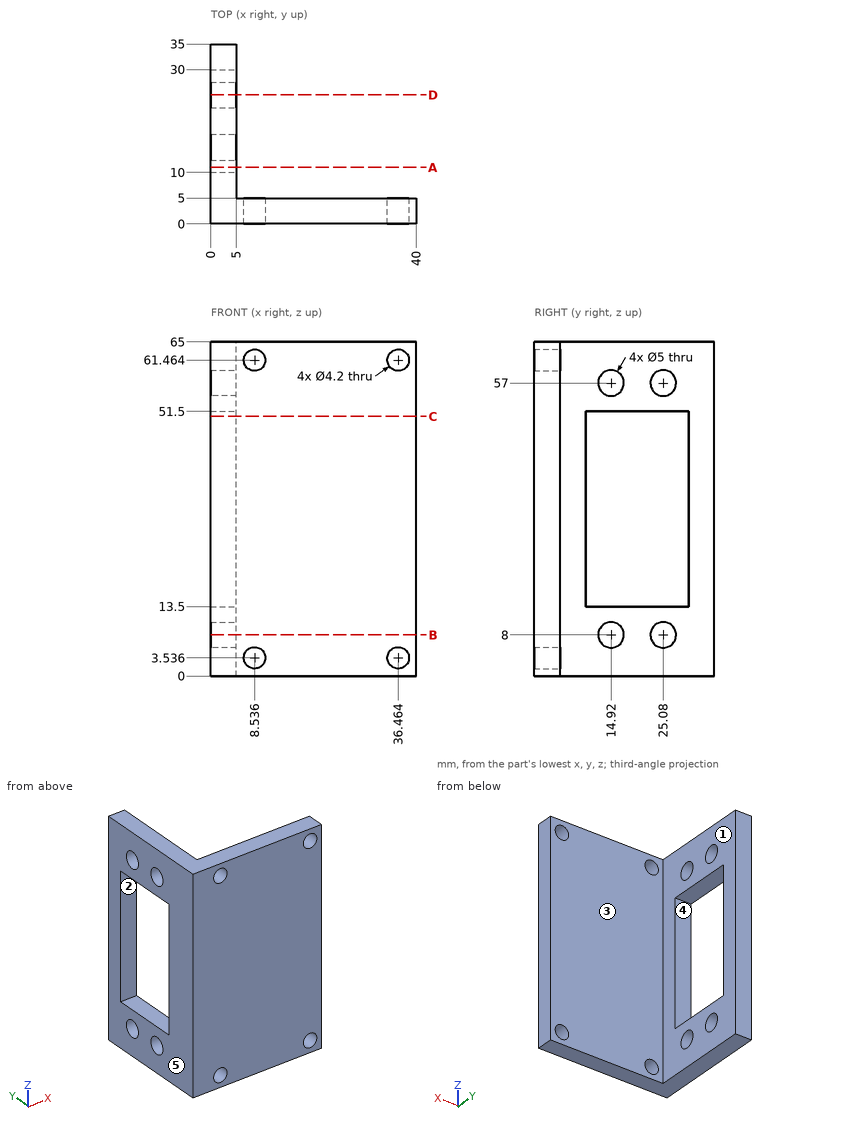
Source: three-view drawing plus pictorial views. Frame: mm from the lowest corner of the part. A direction names the side the tool comes from. Coordinates: 2 decimals unless noted, no trailing zeros. Loops run counter-clockwise (first coordinate to the right, second up) from the corner with the lowest first, then second, coordinate; pieces in that order, holes last. Notation, with made-up numbers: (-38, 8) -> (-17, 8) arc R30 cw to (-17, 41) -> close; hole circle Ø4 at (6, 75.25). An arc over 180 degrees is marked (long way). Write each question's results on one line, items separated by ' | '. Start each with the question number.
Q1. Pull-direction query (Z, two-part tool) for the marked faces 1 and 2; classes: released by +Z, released by -Z, zero draft, split by the parting line, or undercut.
Q2. Section D-D, the plane y = 25.08. Return the cut outline in (x, z).
Q3. Reachability of the marked faces 3, 4 and 5 from +Z, -Z, +X, -X, +Y, -Y: full face, straight path, thin tool, end or side. Return the list, or none.
Q4. Section A-A, the plane y = 11. Return the cut outline in (x, z).
Q5. Section C-C, the plane z = 50.5. Return the cut outline in (x, y), plus the area to 3 significant figures.
Q6. Pin query (flat end, axial travel): pin 1 (4 mm diameter, centred on y = 25.08, z = 57, fed in from +X); pin 2 (15 mm diameter, centred on y = 14.5, z = 31.5, fed in from +X); pin 3 (3 mm diameter, centred on x = 14.5, z = 50.5, fed in from +Y). Return the tip coordinate at first contact, or that it passes through.
Q7. Section B-B, the plane z = 8. Return the cut outline in (x, y), plus the area to 3 significant figures.
Q8. Ray query, line 1 (Y direction, x = 3.45, z = 8); line 2 (Z direction, x = 3, y = 25.5) (1 decimal); line 3 (Y direction, x = 27, z = 51). Return the intervals inside material, ascending. Write a range as from..to.
Found:
1) face 1: zero draft | face 2: undercut
2) outline: (0, 0) -> (5, 0) -> (5, 5.5) -> (0, 5.5) -> close; (0, 10.5) -> (5, 10.5) -> (5, 13.5) -> (0, 13.5) -> close; (0, 51.5) -> (5, 51.5) -> (5, 54.5) -> (0, 54.5) -> close; (0, 59.5) -> (5, 59.5) -> (5, 65) -> (0, 65) -> close
3) face 3: +Z, -Z, +X, +Y | face 4: +X, -X | face 5: +Z, -Z, -X, +Y, -Y
4) outline: (0, 0) -> (5, 0) -> (5, 13.5) -> (0, 13.5) -> close; (0, 51.5) -> (5, 51.5) -> (5, 65) -> (0, 65) -> close
5) outline: (0, 0) -> (40, 0) -> (40, 5) -> (5, 5) -> (5, 10) -> (0, 10) -> close; (0, 30) -> (5, 30) -> (5, 35) -> (0, 35) -> close | area: 250 mm2
6) pin 1: through | pin 2: x = 5 | pin 3: y = 5
7) outline: (0, 0) -> (40, 0) -> (40, 5) -> (5, 5) -> (5, 12.42) -> (0, 12.42) -> close; (0, 17.42) -> (5, 17.42) -> (5, 22.58) -> (0, 22.58) -> close; (0, 27.58) -> (5, 27.58) -> (5, 35) -> (0, 35) -> close | area: 300 mm2
8) line 1: 0..12.42, 17.42..22.58, 27.58..35 | line 2: 0..5.5, 10.5..13.5, 51.5..54.5, 59.5..65 | line 3: 0..5
